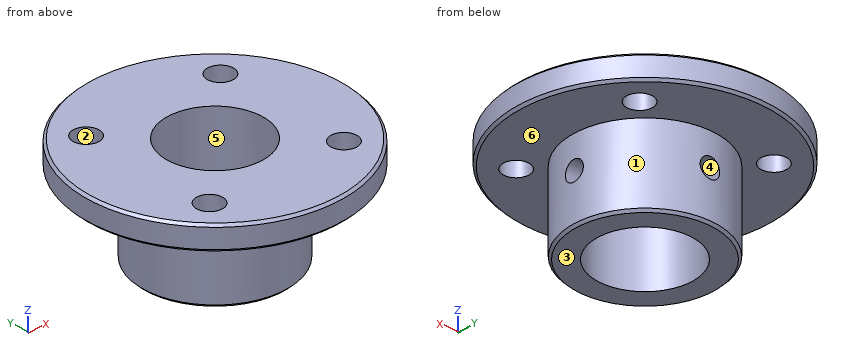
Autodesk Inventor part; units mm, degrees
ref_plane "Work Plane1" through (0, 9, 0) normal (0, 1, 0) x (-1, 0, 0)
ref_plane "Work Plane2" through (9, 0, 0) normal (1, 0, 0) x (0, 1, 0)
ref_plane "XY Plane" through (0, 0, 0) normal (0, 0, 1) x (1, 0, 0)
sketch "Sketch1" plane through (0, 0, 0) normal (1, 0, 0) x (0, 1, 0)
  line L0 (6, 0) -> (16, 0)
  line L1 (16, 0) -> (16, -3)
  line L2 (16, -3) -> (9, -3)
  line L3 (9, -3) -> (9, -13)
  line L4 (9, -13) -> (6, -13)
  line L5 (6, 0) -> (6, -13)
  line L6 (0, -15.6) -> (0, 2.6)
  point P0 (0, 0)
  dimension "d1" = 3
  dimension "d3" = 10
  dimension "d23" = 3
  dimension "d24" = 10
  dimension "d25" = 6
revolve "Revolution1" add sketch "Sketch1" angle 360 about axis through (0, 0, -10) along (0, 0, 1)
chamfer "Chamfer1" distance 0.3 angle 45 3 edges at (0, -16, 0) (0, -16, -3) (0, -9, -13)
sketch "Sketch4" plane through (0, 0, 0) normal (0, 0, 1) x (1, 0, 0)
  line L0 (8.4853, 8.4853) -> (0, 0)
  line L1 (-22.4, 0) -> (22.4, 0)
  point P0 (8.4853, 8.4853)
  dimension "d37" = 45
  dimension "d38" = 8.4853
hole "Hole3" at (8.4853, 8.4853, 0) direction (0, 0, -1) diameter 3.242 depth 6 tip angle 118
pattern_circular "Circular Pattern1" count 4 over 360 about axis through (0, 0, -10) along (0, 0, 1) of "Hole3"
ref_plane "Work Plane1" through (0, 9, 0) normal (0, 1, 0) x (-1, 0, 0)
ref_plane "Work Plane2" through (9, 0, 0) normal (1, 0, 0) x (0, 1, 0)
sketch "Sketch5" plane through (0, 9, 0) normal (0, 1, 0) x (-1, 0, 0)
  line L0 (8.7, -13) -> (-8.7, -13)
  point P0 (0, 0)
  point P1 (0, -7)
  dimension "d41" = 6
sketch "Sketch6" plane through (9, 0, 0) normal (1, 0, 0) x (0, 1, 0)
  line L0 (8.7, -13) -> (-8.7, -13)
  point P0 (0, 0)
  point P1 (0, -7)
  dimension "d42" = 6
hole "Hole4" at (0, 9, -7) direction (0, -1, 0) diameter 2.459 depth 8.8 tip angle 118
hole "Hole5" at (9, 0, -7) direction (-1, 0, 0) diameter 2.459 depth 8.8 tip angle 118
properties part number "kolnierz" material "Iron, Cast"
Geometry check sheet. Reference: the model listing, model coordinates, mm. Face numbers are marked on the shaded views. A direction names the side the tool comes from. Coordinates: 2 decimals unless noted, no trailing zeros. Order: outer loops, then holes, each group sorted by start corner. A loop starts at its lowest first (then second) coordinate and runs counter-clockwise, first axis right, second up. Notation, with made-up numbers: (36, 35.5) - (85, 35.5) arc R17 ccw to (85, 59.5) - close; hole circle Ø8 at (12, 41). An arc over 180 degrees is marked (long way). Answer in a Markdown table with one row per item. Add a question column.
1) Cross-section at D-D, the plane z = -11. Record the cut outline in (x, y), then the cut area to 3 significant figures.
2) Gauge pin test, flat ends, axial feed: P1, Ø5, axis at x = 0, y = 3, coming from the +Z side; P2, Ø3, axis at y = 0, z = -7, coming from the -X side; P3, Ø3, axis at x = -3.5, z = -9.5, coming from the -Y side; P4, Ø10, axis at x = -3.5, y = 12, coming from the -Z side. Record the tip position at first contact, or that the pin passes through.
3) Release check for a two-part mould opening along Y. For the marked faces 1, 2 and 3 record: +Y half, -Y half, draft (parallel to the pull), parting line (faces both ways), or undercut.
4) Cross-section at A-A, the plane x = 0. Record the cut outline in (y, z), then the cut area to 3 significant figures.
5) Set-up check for the marked faces 4, 5 and 6: record each of +Z, -Z, +X, -X, +Y, -Y from which the full face is reachable in a straight line by a thin tool's end or side.
6) Material ranges on line 1 along Y through (x, z) = (0, -11.25); line 2 along Y through (x, z) = (-9.5, -1.25); line 3 along Z through (x, y) = (-1, 10.5), recorded low to high. Write a range as [from, to].
7) Cross-section at C-C, the plane z = -7. Record the cut outline in (x, y), then the cut area to 3 significant figures.
Check result:
| question | item | result |
|---|---|---|
| 1 | outline | circle Ø18 at (0, 0); hole circle Ø12 at (0, 0) |
| 1 | area | 141 mm² |
| 2 | P1 | passes through |
| 2 | P2 | stops at x = -9 |
| 2 | P3 | stops at y = -8.77 |
| 2 | P4 | stops at z = -13 |
| 3 | face 1 | parting line |
| 3 | face 2 | undercut |
| 3 | face 3 | draft |
| 4 | outline | (-16, -2.7) - (-15.7, -3) - (-9, -3) - (-9, -12.7) - (-8.7, -13) - (-6, -13) - (-6, 0) - (-15.7, 0) - (-16, -0.3) - close; (6, -13) - (8.7, -13) - (9, -12.7) - (9, -8.23) - (6, -8.23) - close; (6, -5.77) - (9, -5.77) - (9, -3) - (15.7, -3) - (16, -2.7) - (16, -0.3) - (15.7, 0) - (6, 0) - close |
| 4 | area | 112 mm² |
| 5 | face 4 | +Y |
| 5 | face 5 | +Z, -Z |
| 5 | face 6 | -Z |
| 6 | line 1 | y = [-9, -6], [6, 9] |
| 6 | line 2 | y = [-12.87, -9.75], [-7.22, 7.22], [9.75, 12.87] |
| 6 | line 3 | z = [-3, 0] |
| 7 | outline | (-1.23, 5.87) - (-1.23, 8.92) arc R9 ccw (long way) to (8.92, -1.23) - (5.87, -1.23) arc R6 cw (long way) to start; (1.23, 5.87) arc R6 cw to (5.87, 1.23) - (8.92, 1.23) arc R9 ccw to (1.23, 8.92) - close |
| 7 | area | 127 mm² |
